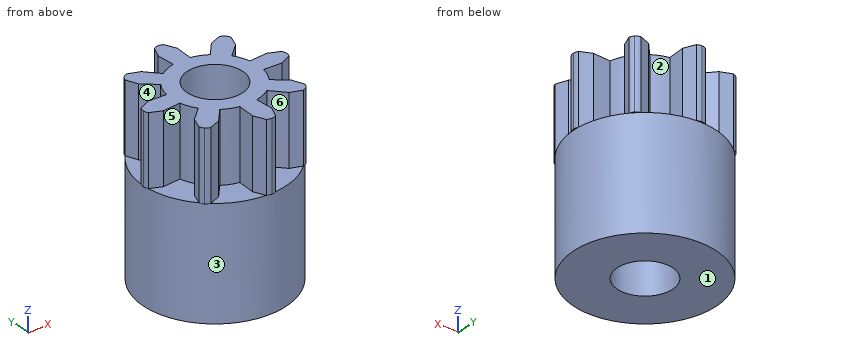
```python
from build123d import *

# Parameters (mm, degrees)
SZKIC1_R                    = 2.5
DODANIE_WYCI_GNI_CIE1_DEPTH = 6.3
SKETCH1_R                   = 6.441701171
SKETCH1_R_2                 = 2.5
BOSS_EXTRUDE1_DEPTH         = 10


with BuildPart() as part:
    # Szkic1 → Dodanie-wyciągnięcie1 (new body)
    with BuildSketch(Plane.XY):
        with BuildLine():
            Line((0.875, 5.423398291), (0.775, 3.822221213))
            ThreePointArc((0.775, 3.822221213), (1.492465386, 3.603130177), (2.154710783, 3.250726294))
            Line((2.154710783, 3.250726294), (3.216203275, 4.453640142))
            Line((3.216203275, 4.453640142), (4.245186445, 4.844987722))
            ThreePointArc((4.245186445, 4.844987722), (4.453444634, 4.765560203), (4.631549417, 4.631549417))
            ThreePointArc((4.631549417, 4.631549417), (4.765560203, 4.453444634), (4.844987722, 4.245186445))
            Line((4.844987722, 4.245186445), (4.453640142, 3.216203275))
            Line((4.453640142, 3.216203275), (3.250726294, 2.154710783))
            ThreePointArc((3.250726294, 2.154710783), (3.603130177, 1.492465386), (3.822221213, 0.775))
            Line((3.822221213, 0.775), (5.423398291, 0.875))
            Line((5.423398291, 0.875), (6.427723795, 0.424123551))
            ThreePointArc((6.427723795, 0.424123551), (6.518820836, 0.220699035), (6.55, 0))
            ThreePointArc((6.55, 0), (6.518820836, -0.220699035), (6.427723795, -0.424123551))
            Line((6.427723795, -0.424123551), (5.423398291, -0.875))
            Line((5.423398291, -0.875), (3.822221213, -0.775))
            ThreePointArc((3.822221213, -0.775), (3.603130177, -1.492465386), (3.250726294, -2.154710783))
            Line((3.250726294, -2.154710783), (4.453640142, -3.216203275))
            Line((4.453640142, -3.216203275), (4.844987722, -4.245186445))
            ThreePointArc((4.844987722, -4.245186445), (4.765560203, -4.453444634), (4.631549417, -4.631549417))
            ThreePointArc((4.631549417, -4.631549417), (4.453444634, -4.765560203), (4.245186445, -4.844987722))
            Line((4.245186445, -4.844987722), (3.216203275, -4.453640142))
            Line((3.216203275, -4.453640142), (2.154710783, -3.250726294))
            ThreePointArc((2.154710783, -3.250726294), (1.492465386, -3.603130177), (0.775, -3.822221213))
            Line((0.775, -3.822221213), (0.875, -5.423398291))
            Line((0.875, -5.423398291), (0.424123551, -6.427723795))
            ThreePointArc((0.424123551, -6.427723795), (0.220699035, -6.518820836), (0, -6.55))
            ThreePointArc((0, -6.55), (-0.220699035, -6.518820836), (-0.424123551, -6.427723795))
            Line((-0.424123551, -6.427723795), (-0.875, -5.423398291))
            Line((-0.875, -5.423398291), (-0.775, -3.822221213))
            ThreePointArc((-0.775, -3.822221213), (-1.492465386, -3.603130177), (-2.154710783, -3.250726294))
            Line((-2.154710783, -3.250726294), (-3.216203275, -4.453640142))
            Line((-3.216203275, -4.453640142), (-4.245186445, -4.844987722))
            ThreePointArc((-4.245186445, -4.844987722), (-4.453444634, -4.765560203), (-4.631549417, -4.631549417))
            ThreePointArc((-4.631549417, -4.631549417), (-4.765560203, -4.453444634), (-4.844987722, -4.245186445))
            Line((-4.844987722, -4.245186445), (-4.453640142, -3.216203275))
            Line((-4.453640142, -3.216203275), (-3.250726294, -2.154710783))
            ThreePointArc((-3.250726294, -2.154710783), (-3.603130177, -1.492465386), (-3.822221213, -0.775))
            Line((-3.822221213, -0.775), (-5.423398291, -0.875))
            Line((-5.423398291, -0.875), (-6.427723795, -0.424123551))
            ThreePointArc((-6.427723795, -0.424123551), (-6.518820836, -0.220699035), (-6.55, 0))
            ThreePointArc((-6.55, 0), (-6.518820836, 0.220699035), (-6.427723795, 0.424123551))
            Line((-6.427723795, 0.424123551), (-5.423398291, 0.875))
            Line((-5.423398291, 0.875), (-3.822221213, 0.775))
            ThreePointArc((-3.822221213, 0.775), (-3.603130177, 1.492465386), (-3.250726294, 2.154710783))
            Line((-3.250726294, 2.154710783), (-4.453640142, 3.216203275))
            Line((-4.453640142, 3.216203275), (-4.844987722, 4.245186445))
            ThreePointArc((-4.844987722, 4.245186445), (-4.765560203, 4.453444634), (-4.631549417, 4.631549417))
            ThreePointArc((-4.631549417, 4.631549417), (-4.453444634, 4.765560203), (-4.245186445, 4.844987722))
            Line((-4.245186445, 4.844987722), (-3.216203275, 4.453640142))
            Line((-3.216203275, 4.453640142), (-2.154710783, 3.250726294))
            ThreePointArc((-2.154710783, 3.250726294), (-1.492465386, 3.603130177), (-0.775, 3.822221213))
            Line((-0.775, 3.822221213), (-0.875, 5.423398291))
            Line((-0.875, 5.423398291), (-0.424123551, 6.427723795))
            ThreePointArc((-0.424123551, 6.427723795), (-0.220699035, 6.518820836), (0, 6.55))
            ThreePointArc((0, 6.55), (0.220699035, 6.518820836), (0.424123551, 6.427723795))
            Line((0.424123551, 6.427723795), (0.875, 5.423398291))
        make_face()
        Circle(SZKIC1_R, mode=Mode.SUBTRACT)
    extrude(amount=DODANIE_WYCI_GNI_CIE1_DEPTH)

    # Sketch1 → Boss-Extrude1 (add)
    with BuildSketch(Plane.XY):
        Circle(SKETCH1_R)
        Circle(SKETCH1_R_2, mode=Mode.SUBTRACT)
    extrude(amount=-BOSS_EXTRUDE1_DEPTH)


solid = part.part
```
The listing builds one solid part. Answer for the finished solid, in the listing's coordinates (mm). Face numbers are marked on the shaded views. A direction names the side the tool comes from. Coordinates: 2 decimals unless noted, no trailing zeros. Write each loop counter-clockwise with the first axis right and the second up, starting at its lowest first coordinate (ties: lowest second). Pieces come first, ordered by that corner, then holes. Notation, with made-up numbers: M 65,59 L 75,59 A20 ccw 75,86 Z; hole C -40,66 d6. An arc over 180 degrees is marked long. Use a Markdown table: item, result. Add a question column.
1. Section B-B (y = 1.25) is taken. Give the vertices of the cut face in (x, z).
2. Given P1, Ø3.5, axis at x = -5.5, y = 2, coming from the +Z side; P2, Ø4, axis at y = -3, z = -6, coming from the -X side; P3, Ø1.6, axis at x = -5, y = -2, coming from the +Z side; P4, Ø1.5, axis at x = -2, z = -8, coming from the -Y side, each flat-ended and moving along its own axis, determine where each tip first touches the part or whether it passes through.
3. Straight lines are drawn through the part: line 1 along Y through (x, z) = (0, -4); line 2 along Z through (x, y) = (4.5, 2.75); line 3 along Y through (x, z) = (1.5, -4.75). For each, find the intervals that lie inside material, in ascending order. Write a range as [from, to].
4. Section C-C (z = -8.5) is taken. Give the vertices of the cut face in (x, y).
5. Which of the six approach directions +Z, -Z, +X, -X, +Y, -Y give full straight-line access (tool end or side, diameter ignored) to the marked faces 4, 5 and 6?
6. For a pull along X with two mould halves and no side action, classify the marked faces 1, 2 and 3 as +X half, -X half, draft (parallel to the pull), parting line (faces both ways), or undercut.
7. Section A-A (x = -1.5) is taken. Give the vertices of the cut face in (y, z), plus the area to 3 significant figures.
Data:
| question | item | result |
|---|---|---|
| 1 | outline | M -6.32,-10 L -2.17,-10 L -2.17,6.3 L -3.69,6.3 L -3.69,0 L -6.32,0 Z; M 2.17,-10 L 6.32,-10 L 6.32,0 L 3.69,0 L 3.69,6.3 L 2.17,6.3 Z |
| 2 | P1 | stops at z = 6.3 |
| 2 | P2 | stops at x = -6.36 |
| 2 | P3 | stops at z = 0 |
| 2 | P4 | stops at y = -6.32 |
| 3 | line 1 | y = [-6.44, -2.5], [2.5, 6.44] |
| 3 | line 2 | z = [-10, 0] |
| 3 | line 3 | y = [-6.26, -2], [2, 6.26] |
| 4 | outline | C 0,0 d12.88; hole C 0,0 d5 |
| 5 | face 4 | +Z, -X |
| 5 | face 5 | +Z |
| 5 | face 6 | +Z, -Y |
| 6 | face 1 | draft |
| 6 | face 2 | undercut |
| 6 | face 3 | parting line |
| 7 | outline | M -6.26,-10 L -2,-10 L -2,6.3 L -3.6,6.3 L -3.6,0 L -6.26,0 Z; M 2,-10 L 6.26,-10 L 6.26,0 L 3.6,0 L 3.6,6.3 L 2,6.3 Z |
| 7 | area | 105 mm2 |
